For this review, take the finished solid that the model builds, in its own axes (mm). A direction names the side the tool comes from. Round coordinates to 2 decimals unless told otherwise and drop trailing zeros. Write each loop counter-clockwise with the first axis right and the second up, starting at its lowest first coordinate (ties: lowest second). Pieces come first, ordered by that corner, then holes. Notation, with made-up numbers: (-8.5, -23) -> (20.5, -23) arc R16 cw to (20.5, -19) -> close; hole circle Ø4 at (-6.5, 50). An arc over 180 degrees is marked (long way). Answer as CSV lines item,"result". Start each with the question number.
Item 1: Take a section at B-B on y = 88. Give the boundary of the cut face in (x, z).
Item 2: For pin 1 Ø10 at (y, z) = (12, -61.5) entering from +X; pin 2 Ø1.5 at (x, y) = (-65.5, 57) entering from -Z; pin 3 Ø4 at (x, z) = (-50, -28) entering from -Y, all flat-tipped, find the tip position at first contact; note any pin that passes through.
Item 3: Wall thickness on probe 1 along Y at (x, z) = (-32, -62); probe 2 along Y at (x, z) = (-4, -83.5); probe 3 along X at (y, z) = (8.5, -73.5): over which ranges is each line inside the solid? List them lowest first. Write a range as from..to.
Item 4: Mouldability with a two-part tool opening along Y and no side actions: class faces 1 (the flat face through (-49, 98, -100)), 2 (the flat face through (-76, 0, -51)), 3 (the flat face through (-91.5, 93, -56)) as +Y half, -Y half, draft (parallel to the pull), parting line (faces both ways), or undercut.
Item 5: Take a section at A-A on x = -37.5. Give the boundary of the cut face in (y, z).
Item 6: Machinability: for faces 4 (the flat face through (-3.5, 5, -56)), 5 (the flat face through (-97.5, 51, -5)), 6 (the flat face through (-93, 10, -51)), which of the approach directions +Z, -Z, +X, -X, +Y, -Y give a long, thin tool a straight path to every point of the face, cutting with its end or side? Answer none if there is none.
Autodesk Inventor part; units mm, degrees
ref_plane "Work Plane1" through (-3.4, 0, -10.1) normal (0, 0, 1) x (1, 0, 0)
ref_plane "YZ Plane" through (0, 0, 0) normal (1, 0, 0) x (0, 1, 0)
ref_plane "XZ Plane" through (0, 0, 0) normal (0, 1, 0) x (-1, 0, 0)
sketch "Sketch1" plane through (0, 0, 0) normal (1, 0, 0) x (0, 1, 0)
  line L0 (0, 0) -> (100, 0)
  line L1 (100, 0) -> (100, -100)
  line L2 (100, -100) -> (90, -100)
  line L3 (90, -100) -> (90, -10)
  line L4 (90, -10) -> (10, -10)
  line L5 (10, -10) -> (10, -100)
  line L6 (10, -100) -> (0, -100)
  line L7 (0, -100) -> (0, 0)
  dimension "d0" = 100
  dimension "d1" = 100
  dimension "d2" = 10
  dimension "d3" = 10
  dimension "d4" = 10
extrude "Extrusion1" add sketch "Sketch1" against normal blind 100
sketch "Sketch2" plane through (0, 90, -100) normal (0, 0, -1) x (-1, 0, 0)
  line L0 (50, -90) -> (50, 10) construction
  line L1 (0, -40) -> (100, -40) construction
  line L2 (100, 0) -> (100, -80)
  line L3 (0, -90) -> (100, -90)
  line L4 (0, 10) -> (100, 10)
  line L5 (1, 10) -> (1, 7.5)
  line L6 (1, 7.5) -> (3.5, 9)
  line L7 (3.5, 9) -> (3.5, 1)
  line L8 (3.5, 1) -> (1, 2.5)
  line L9 (1, 2.5) -> (1, -40)
  line L10 (0, 0) -> (0, 10)
  line L11 (99, 10) -> (99, 7.5)
  line L12 (99, 7.5) -> (96.5, 9)
  line L13 (96.5, 9) -> (96.5, 1)
  line L14 (96.5, 1) -> (99, 2.5)
  line L15 (99, 2.5) -> (99, -40)
  line L16 (100, 0) -> (100, 10)
  line L17 (0, -90) -> (100, -90)
  line L18 (1, -90) -> (1, -87.5)
  line L19 (1, -87.5) -> (3.5, -89)
  line L20 (3.5, -89) -> (3.5, -81)
  line L21 (3.5, -81) -> (1, -82.5)
  line L22 (1, -82.5) -> (1, -40)
  line L23 (0, -80) -> (0, -90)
  line L24 (99, -82.5) -> (99, -40)
  line L25 (96.5, -81) -> (99, -82.5)
  line L26 (96.5, -89) -> (96.5, -81)
  line L27 (99, -87.5) -> (96.5, -89)
  line L28 (100, -80) -> (100, -90)
  line L29 (99, -90) -> (99, -87.5)
  line L30 (0, 10) -> (100, 10)
  line L31 (100, 10) -> (100, -90)
  line L32 (100, -90) -> (0, -90)
  line L33 (0, -90) -> (0, 10)
  point P0 (50, -40)
  dimension "d12" = 2.5
  dimension "d14" = 8
  dimension "d15" = 2.5
  dimension "d16" = 1
  dimension "d18" = 1
  dimension "d19" = 59.036
extrude "Extrusion2" cut sketch "Sketch2" against normal blind 90 contours L2 L28 L3 L29 L27 L26 L25 L24 L15 L14 L13 L12 L11 L4 L16 | L5 L6 L7 L8 L9 L22 L21 L20 L19 L18 L3 L23 L33 L10 L4
sketch "Sketch3" plane through (0, 100, 0) normal (0, 1, 0) x (1, 0, 0)
  line L0 (0, 0) -> (0, 10)
  line L1 (0, 0) -> (0, 2.5)
  line L2 (0, 2.5) -> (2.5, 1)
  line L3 (2.5, 1) -> (2.5, 9)
  line L4 (2.5, 9) -> (0, 7.5)
  line L5 (0, 10) -> (0, 0)
  line L6 (-1, 10) -> (0, 10)
  line L7 (0, 10) -> (0, 7.5)
  line L8 (0, 0) -> (-100, 0)
  line L9 (-97.5, 1) -> (-97.5, 9)
  line L10 (-97.5, 9) -> (-100, 7.5)
  line L11 (-100, 0) -> (-100, 10)
  line L12 (-100, 7.5) -> (-100, 2.5)
  line L13 (-97.5, 1) -> (-100, 2.5)
  dimension "d22" = 2.5
  dimension "d23" = 2.5
  dimension "d24" = 8
  dimension "d25" = 2.5
  dimension "d26" = 1
  dimension "d27" = 2.5
  dimension "d28" = 2.5
  dimension "d29" = 8
  dimension "d30" = 2.5
  dimension "d31" = 1
extrude "Extrusion3" add sketch "Sketch3" against normal up to surface (100 mm away) contours L0 L4 L3 L2
extrude "Extrusion4" cut sketch "Sketch3" against normal up to surface (100 mm away) contours L11 L10 L9 L13
sketch "Sketch4" plane through (-1, 90, -100) normal (0, 0, -1) x (-1, 0, 0)
  line L0 (0, -90) -> (98, -90)
  line L1 (46.5, -90) -> (45, -87.5)
  line L2 (45, -87.5) -> (53, -87.5)
  line L3 (53, -87.5) -> (51.5, -90)
  line L4 (0, 10) -> (98, 10)
  line L5 (49, 10) -> (49, -90) construction
  line L6 (46.5, -90) -> (51.5, -90)
  line L7 (45, 12.5) -> (53, 12.5)
  line L8 (53, 12.5) -> (51.5, 10)
  line L9 (42.8887, 10) -> (51.5, 10)
  line L10 (45, 12.5) -> (46.5, 10)
  line L11 (51.5, 10) -> (46.5, 10)
  point P0 (-1, -90)
  point P1 (49, -87.5)
  point P2 (49, -40)
  point P3 (49, -90)
  point P4 (49, 12.5)
  dimension "d36" = 8
  dimension "d37" = 2.5
  dimension "d38" = 5
  dimension "d39" = 2.5
  dimension "d40" = 8
  dimension "d42" = 5
extrude "Extrusion5" add sketch "Sketch4" against normal up to surface (100 mm away) contours L10 L7 L8 L4
extrude "Extrusion6" cut sketch "Sketch4" against normal up to surface (100 mm away) contours L1 L2 L3 L0
sketch "Sketch7" plane through (-1, 90, -100) normal (1, 0, 0) x (0, 0, -1)
  line L0 (0, 10) -> (0, 7.5)
  line L1 (-90, -87.5) -> (-90, -90)
  line L2 (0, 10) -> (-90, 10)
  line L3 (-90, 10) -> (-90, -90)
  line L4 (-90, -90) -> (0, -90)
  line L5 (0, -90) -> (0, 10)
  point P0 (-100, -90)
extrude "Extrusion9" cut sketch "Sketch7" against normal blind 0.1
sketch "Sketch8" plane through (-96.5, 91, -100) normal (0, 0, -1) x (-1, 0, 0)
  line L0 (-96.5, 9) -> (-49, 9)
  line L1 (-42.5, 11.5) -> (-50.5, 11.5)
  line L2 (-49, 9) -> (-50.5, 11.5)
  line L3 (-50.5, 11.5) -> (-42.5, 11.5)
  line L4 (-44, 9) -> (-42.5, 11.5)
  line L5 (-42.5, 11.5) -> (-44, 9)
  line L6 (-49, 9) -> (-44, 9)
  line L7 (-42.6766, 11.4) -> (-44.1166, 9)
  line L8 (-50.3234, 11.4) -> (-48.8834, 9)
  line L9 (-50.3234, 11.4) -> (-42.6766, 11.4)
  point P0 (-96.5, -91)
  dimension "d59" = 0.1
  dimension "d60" = 0.1
  dimension "d61" = 0.1
extrude "Extrusion10" cut sketch "Sketch8" against normal up to surface (100 mm away) contours L4 L6 L7 L9 L8 L2 L1
sketch "Sketch9" plane through (-99, 97.5, -100) normal (-1, 0, 0) x (0, 0, 1)
  line L0 (0, 2.5) -> (90, 2.5)
  line L1 (90, 2.5) -> (90, -97.5)
  line L2 (0, 2.5) -> (90, 2.5)
  line L3 (90, 2.5) -> (90, -97.5)
  line L4 (90, -97.5) -> (0, -97.5)
  line L5 (0, -97.5) -> (0, 2.5)
  point P0 (100, -97.5)
extrude "Extrusion11" cut sketch "Sketch9" against normal blind 0.1
sketch "Sketch10" plane through (2.5, 100, -1) normal (0, 1, 0) x (1, 0, 0)
  line L0 (0, 8) -> (-2.5, 6.5)
  line L1 (-2.5, 6.5) -> (0, 8)
  line L2 (-2.5, 1.5) -> (0, 0)
  line L3 (0, 8) -> (0, 0)
  line L4 (0, 0) -> (-2.5, 1.5)
  line L5 (-2.5, 6.3834) -> (-0.1, 7.8234)
  line L6 (-0.1, 7.8234) -> (-0.1, 0.1766)
  line L7 (-0.1, 0.1766) -> (-2.5, 1.6166)
  line L8 (0, 8) -> (-2.5, 6.5)
  line L9 (-2.5, 6.5) -> (-2.5, 9)
  line L10 (-2.5, 6.5) -> (-2.5, 1.5)
  point P0 (-2.5, -1)
  dimension "d66" = 0.1
  dimension "d67" = 0.1
  dimension "tol" = 0.1
extrude "Extrusion12" cut sketch "Sketch10" against normal through all contours L3 L2 L10 L7 L6 L5 L0
sketch "Sketch11" plane through (-3.5, 91, -100) normal (0, 0, -1) x (-1, 0, 0)
  line L0 (-2.4, -1) -> (95.4, -1)
  line L1 (5, -1) -> (88, -1)
  line L2 (88, -1) -> (88, 6)
  line L3 (88, 6) -> (5, 6)
  line L4 (5, 6) -> (5, -1)
  line L5 (0, 8) -> (0, 0)
  line L6 (93, 0) -> (93, 8)
  line L7 (48.8834, 9) -> (95.4, 9)
  point P0 (-3.5, -91)
  point P1 (88, -1)
  dimension "d71" = 5
  dimension "d72" = 5
  dimension "d73" = 3
ref_plane "Work Plane1" through (-3.4, 0, -10.1) normal (0, 0, 1) x (1, 0, 0)
extrude "Extrusion13" cut sketch "Sketch11" against normal up to surface (89.9 mm away)
ref_plane "Work Plane2" through (-1.1, 50, -10) normal (0, 1, 0) x (1, 0, 0)
mirror "Mirror1" about plane through (-1.1, 50, -10) normal (0, 1, 0) of "Extrusion13"
equation "\"d54\" = tol"
equation "\"d59\" = tol"
equation "\"d60\" = tol"
equation "\"d61\" = tol"
equation "\"d64\" = tol"
equation "\"d66\" = tol"
equation "\"d67\" = tol"
properties part number "mainframe"
Output values:
1,outline,"(-100, -10) -> (0, -10) -> (0, -7.38) -> (2.4, -8.82) -> (2.4, -1.18) -> (0, -2.62) -> (0, 0) -> (-100, 0) -> (-100, -2.5) -> (-97.5, -1) -> (-97.5, -9) -> (-100, -7.5) -> close"
2,pin 1,"stops at x = -1.1"
2,pin 2,"stops at z = -10"
2,pin 3,"stops at y = 2.5"
3,probe 1,"y = 0..3, 97..100"
3,probe 2,"y = 0..10, 90..100"
3,probe 3,"x = -98.9..-97.33, -96.5..-91.5, -8.5..-3.5, -2.67..-1.1"
4,face 1,"draft"
4,face 2,"-Y half"
4,face 3,"undercut"
5,outline,"(0, -100) -> (3, -100) -> (3, -10.1) -> (10, -10.1) -> (10, -10) -> (90, -10) -> (90, -10.1) -> (97, -10.1) -> (97, -100) -> (100, -100) -> (100, 0) -> (0, 0) -> close"
6,face 4,"-Z"
6,face 5,"+Y, -Y"
6,face 6,"-Z, +X, -X"
